Here's how the part is built. I have some questions about the finished solid (model axes, mm). Face numbers are marked on the shaded views. A direction names the side the tool comes from. Round coordinates to 2 decimals unless told otherwise and drop trailing zeros. Order: outer loops, then holes, each group sorted by start corner. A loop starts at its lowest first (then second) coordinate and runs counter-clockwise, first axis right, second up. Notation, with made-up numbers: (-35.5, 22) -> (-13.5, 22) arc R6 cw to (-13.5, 27) -> close; hole circle Ø2 at (64, 64). An arc over 180 degrees is marked (long way). Answer in a Markdown table with one row per item.
```python
from build123d import *

# Parameters (mm, degrees)
CROQUIS2_R              = 2
SALIENTE_EXTRUIR1_DEPTH = 8
CROQUIS3_R              = 2
SALIENTE_EXTRUIR2_DEPTH = 8
REDONDEO1_R             = 0.03
REDONDEO2_R             = 0.03


with BuildPart() as part:
    # Croquis1 → Revolución1 (revolve)
    with BuildSketch(Plane.XY, mode=Mode.PRIVATE) as revoluci_n1_sk:
        Polygon((0, 0), (0, 2), (4, 2), (4, 8), (11.5, 8), (11.5, 5), (24, 5), (24, 2), (28, 2), (28, 0), align=None)
    revolve(revoluci_n1_sk.sketch.rotate(Axis((0, 0, 0), (1, 0, 0)), 90), axis=Axis((0, 0, 0), (1, 0, 0)))

    # Croquis2 → Saliente-Extruir1 (add)
    with BuildSketch(Plane.ZY):
        Circle(CROQUIS2_R)
    extrude(amount=SALIENTE_EXTRUIR1_DEPTH)

    # Croquis3 → Saliente-Extruir2 (add)
    with BuildSketch(Plane(origin=(28, 0, 0), x_dir=(0, 0, -1), z_dir=(1, 0, 0))):
        with Locations(Location((0, 0, 0), (0, 0, 180))):
            Circle(CROQUIS3_R)
    extrude(amount=SALIENTE_EXTRUIR2_DEPTH)

    # Redondeo1
    redondeo1_edges = [part.edges().sort_by_distance(p)[0] for p in [
        (4, 0, -2),
    ]]
    fillet(redondeo1_edges, radius=REDONDEO1_R)

    # Redondeo2
    redondeo2_edges = [part.edges().sort_by_distance(p)[0] for p in [
        (11.5, 0, -5),
        (24, 0, -2),
    ]]
    fillet(redondeo2_edges, radius=REDONDEO2_R)


solid = part.part
```
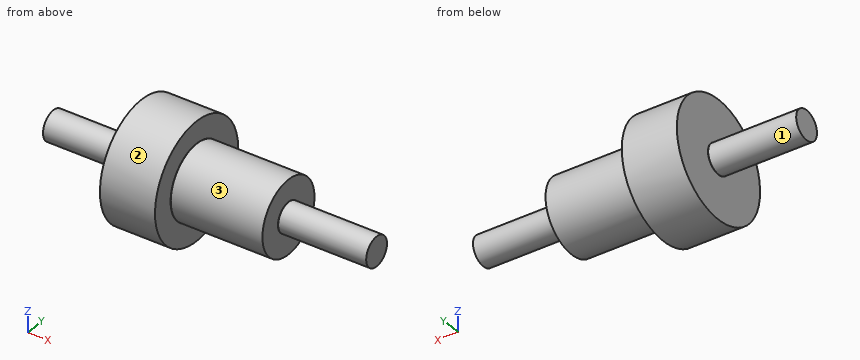
1. Suppose I cut it at C-C on x = 30. Write out the boundary of the cut face in (y, z).
Numbers:
| item | result |
|---|---|
| outline | circle Ø4 at (0, 0) |
2. For pin 1 Ø5 at (x, y) = (-0.5, 2.5) entering from -Z; pin 2 Ø1 at (x, z) = (15.5, 3.5) entering from +Y; pin 3 Ø5 at (x, y) = (25.5, 4.5) entering from -Z, each with a flat end and sliding along its axis, tell me the tip position at first contact or that it passes through.
Numbers:
| item | result |
|---|---|
| pin 1 | stops at z = -2 |
| pin 2 | stops at y = 4 |
| pin 3 | stops at z = -4.33 |
3. Suppose I cut it at D-D on z = -5.75. Write out the boundary of the cut face in (x, y), then the cut area to 3 significant figures.
Numbers:
| item | result |
|---|---|
| outline | (4, -5.56) -> (11.5, -5.56) -> (11.5, 5.56) -> (4, 5.56) -> close |
| area | 83.4 mm2 |
4. Please list where these lines run through material, in increasing order: line 1 along X through (y, z) = (-4.5, -2); line 2 along X through (y, z) = (3.75, 4.75); line 3 along Z through (x, y) = (19.5, 4).
Numbers:
| item | result |
|---|---|
| line 1 | x = 4 to 24 |
| line 2 | x = 4 to 11.5 |
| line 3 | z = -3 to 3 |
5. Suppose I cut it at A-A on z = 0. Write out the boundary of the cut face in (x, y), then the cut area to 3 significant figures.
Numbers:
| item | result |
|---|---|
| outline | (-8, -2) -> (3.97, -2) arc R0.03 cw to (4, -2.03) -> (4, -8) -> (11.5, -8) -> (11.5, -5.03) arc R0.03 cw to (11.53, -5) -> (24, -5) -> (24, -2.03) arc R0.03 cw to (24.03, -2) -> (36, -2) -> (36, 2) -> (24.03, 2) arc R0.03 cw to (24, 2.03) -> (24, 5) -> (11.53, 5) arc R0.03 cw to (11.5, 5.03) -> (11.5, 8) -> (4, 8) -> (4, 2.03) arc R0.03 cw to (3.97, 2) -> (-8, 2) -> close |
| area | 341 mm2 |
6. For the marked faces 1, 2 and 3, which set-ups out of +Z, -Z, +X, -X, +Y, -Y let a thin tool reach every point of the face, with its end or its side?
Numbers:
| item | result |
|---|---|
| face 1 | -X |
| face 2 | +X, -X |
| face 3 | +X |
